The model under review builds one solid part; all positions refer to its coordinate system, in mm. A direction names the side the tool comes from. Give positions to 0.01 mm unless a question says otherwise; leave off trailing zeros. Order: outer loops, then holes, each group sorted by start corner. A loop starts at its lowest first (then second) coordinate and runs counter-clockwise, first axis right, second up.
```python
from build123d import *

# Parameters (mm, degrees)
BOSS_EXTRUDE2_DEPTH = 16.8
SKETCH5_R           = 3.65
CUT_EXTRUDE3_DEPTH  = 28.5


with BuildPart() as part:
    # Sketch1 → Boss-Extrude2 (new body)
    with BuildSketch(Plane(origin=(0, 0, 0), x_dir=(1, 0, 0), z_dir=(0, 1, 0))):
        Polygon((2.5, -9.25), (-2.5, -9.25), (-57.5, -9.25), (-57.5, -14.25), (2.5, -14.25), align=None)
        Polygon((2.5, 9.25), (-2.5, 9.25), (-2.5, 4.25), (-2.5, -9.25), (2.5, -9.25), align=None)
        Polygon((-57.5, 9.25), (-2.5, 9.25), (2.5, 9.25), (2.5, 14.25), (-57.5, 14.25), align=None)
    extrude(amount=-BOSS_EXTRUDE2_DEPTH)

    # Sketch5 → Cut-Extrude3 (cut)
    with BuildSketch(Plane.XY.offset(14.25)):
        with Locations((-47.5, -8.4)):
            Circle(SKETCH5_R)
    extrude(amount=-CUT_EXTRUDE3_DEPTH, mode=Mode.SUBTRACT)


solid = part.part
```
1. For faces 4 (the flat face through (2.5, -8, 0)), 5 (the flat face through (-30, -8, 9.25)), list the 3-axis set-ups (+Z, -Z, +X, -X, +Y, -Y) from which the entire face can be reached by the end or side of a thin tool; tool diameter is ignored.
2. Take a section at C-C (x = -47.5). Write out the cut boundary in (y, z), and give its area (3 significant figures).
3. To check wall thickness, follow line 1 (Z direction, x = -37, y = -2); line 2 (Y direction, x = -47.5, z = 11.8); line 3 (X direction, y = -8, z = -8.75). State the ranges of each line that lie inside material, in increasing order.
4. Insertion check: pin 1 (5 mm diameter, centred on y = -9, z = 1, fed in from -X). The pin has a flat end and moves straight along its axis. Give the tip position at first contact, or say it passes through.
5. Take a section at B-B (y = -6). Write out the cut boundary in (x, z).
6. Take a section at A-A (x = -30). Write out the cut boundary in (y, z).
7. Take a section at D-D (y = -2.75). Write out the cut boundary in (x, z).
8. Draft analysis for pull direction Z (two halves, no side actions). For faces 1 (the cylindrical face through (-50.19, -5.93, 11.78)), 2 (the flat face through (-30, -8, -9.25)), 3 (the flat face through (-28, -8, 14.25)), state which applies: pulls with the +Z half, pulls with the -Z half, needs draft (parallel to the pull), parting line crosses it, or undercut.
Answer:
1. face 4: +Z, -Z, +X, +Y, -Y
1. face 5: -X, +Y, -Y
2. outline: (-16.8, -14.25) - (-12.05, -14.25) - (-12.05, -9.25) - (-16.8, -9.25) - close; (-16.8, 9.25) - (-12.05, 9.25) - (-12.05, 14.25) - (-16.8, 14.25) - close; (-4.75, -14.25) - (0, -14.25) - (0, -9.25) - (-4.75, -9.25) - close; (-4.75, 9.25) - (0, 9.25) - (0, 14.25) - (-4.75, 14.25) - close
2. area: 95.0 mm2
3. line 1: z = -14.25 to -9.25, 9.25 to 14.25
3. line 2: y = -16.8 to -12.05, -4.75 to 0
3. line 3: x = -2.5 to 2.5
4. pin 1: stops at x = -2.5
5. outline: (-57.5, -14.25) - (-50.25, -14.25) - (-50.25, -9.25) - (-57.5, -9.25) - close; (-57.5, 9.25) - (-50.25, 9.25) - (-50.25, 14.25) - (-57.5, 14.25) - close; (-44.75, -14.25) - (2.5, -14.25) - (2.5, 14.25) - (-44.75, 14.25) - (-44.75, 9.25) - (-2.5, 9.25) - (-2.5, -9.25) - (-44.75, -9.25) - close
6. outline: (-16.8, -14.25) - (0, -14.25) - (0, -9.25) - (-16.8, -9.25) - close; (-16.8, 9.25) - (0, 9.25) - (0, 14.25) - (-16.8, 14.25) - close
7. outline: (-57.5, -14.25) - (2.5, -14.25) - (2.5, 14.25) - (-57.5, 14.25) - (-57.5, 9.25) - (-2.5, 9.25) - (-2.5, -9.25) - (-57.5, -9.25) - close
8. face 1: needs draft
8. face 2: undercut
8. face 3: pulls with the +Z half
